Geometry check sheet. Reference: the model listing, model coordinates, mm. Face numbers are marked on the shaded views. A direction names the side the tool comes from. Coordinates: 2 decimals unless noted, no trailing zeros. Order: outer loops, then holes, each group sorted by start corner. A loop starts at its lowest first (then second) coordinate and runs counter-clockwise, first axis right, second up. Notation, with made-up numbers: M 1,1 L 25,1 A32 cw 25,40 Z; hole C 77,13.25 d1. An arc over 180 degrees is marked long. One line per item, written item: value. Start each with the question number.
1) Thickness scan on L1, parallel to Y at x = 132, z = 92; L2, parallel to Z at x = 136.5, y = 218. Record the ranges inside material, lowest first. Write a range as from..to.
2) Sectioned sample at C-C, the plane z = 78.5. Enter the section's corners in (x, y).
3) Access from +Z, -Z, +X, -X, +Y, -Y to the whole of each face (thin tool, end or side, straight path). Record for the marked faces 1 and 2.
4) Go/stop test with flat-tipped pins: P1, Ø15.5, axis at x = 66, z = 80.5, coming from the +Y side; P2, Ø17.5, axis at x = 101, y = 197, coming from the +Z side. Record where each tip stops, or that it passes through.
5) Sectioned sample at B-B, the plane y = 205. Enter the section's corners in (x, z), then the cut area to 3 significant figures.
6) Sectioned sample at A-A, the plane x = 124. Enter the section's corners in (y, z).
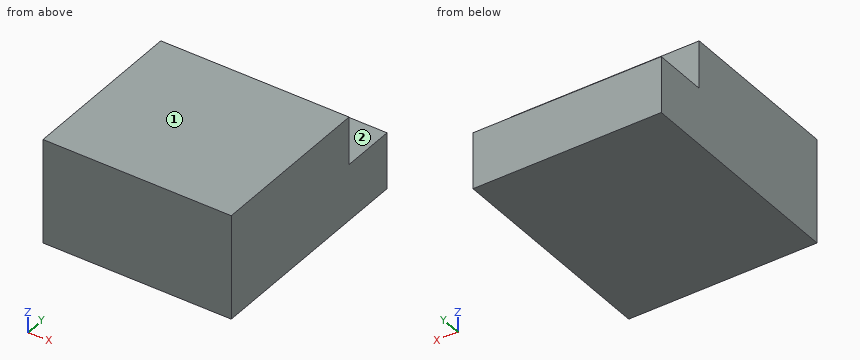
Autodesk Inventor part; units mm, degrees
ref_plane "Plan YZ" through (0, 0, 0) normal (1, 0, 0) x (0, 1, 0)
ref_plane "Plan XZ" through (0, 0, 0) normal (0, 1, 0) x (-1, 0, 0)
ref_plane "Plan XY" through (0, 0, 0) normal (0, 0, 1) x (1, 0, 0)
sketch "Esquisse1" plane through (0, 0, 0) normal (0, 0, 1) x (1, 0, 0)
  line L0 (0, 0) -> (200, 0)
  line L1 (200, 0) -> (200, 238)
  line L2 (200, 238) -> (0, 238)
  line L3 (0, 238) -> (0, 0)
  line L4 (0, 0) -> (200, 0)
  line L5 (200, 0) -> (200, 180)
  line L6 (200, 180) -> (0, 180)
  line L7 (0, 180) -> (0, 0)
  point P0 (0, 180)
  dimension "d0" = 200
  dimension "d1" = 238
  dimension "d2" = 180
extrude "Extrusion1" add sketch "Esquisse1" along normal blind 111 contours L3 L6 L1 L0
extrude "Extrusion2" add sketch "Esquisse1" along normal blind 60 contours L3 L2 L1 L6
properties part number "coffretElec"
Final values:
1. L1: y = 0..180
1. L2: z = 0..60
2. outline: M 0,0 L 200,0 L 200,180 L 0,180 Z
3. face 1: +Z, +X, -X, +Y, -Y
3. face 2: +Z, +X, -X, +Y
4. P1: stops at y = 180
4. P2: stops at z = 60
5. outline: M 0,0 L 200,0 L 200,60 L 0,60 Z
5. area: 12,000 mm^2
6. outline: M 0,0 L 238,0 L 238,60 L 180,60 L 180,111 L 0,111 Z
